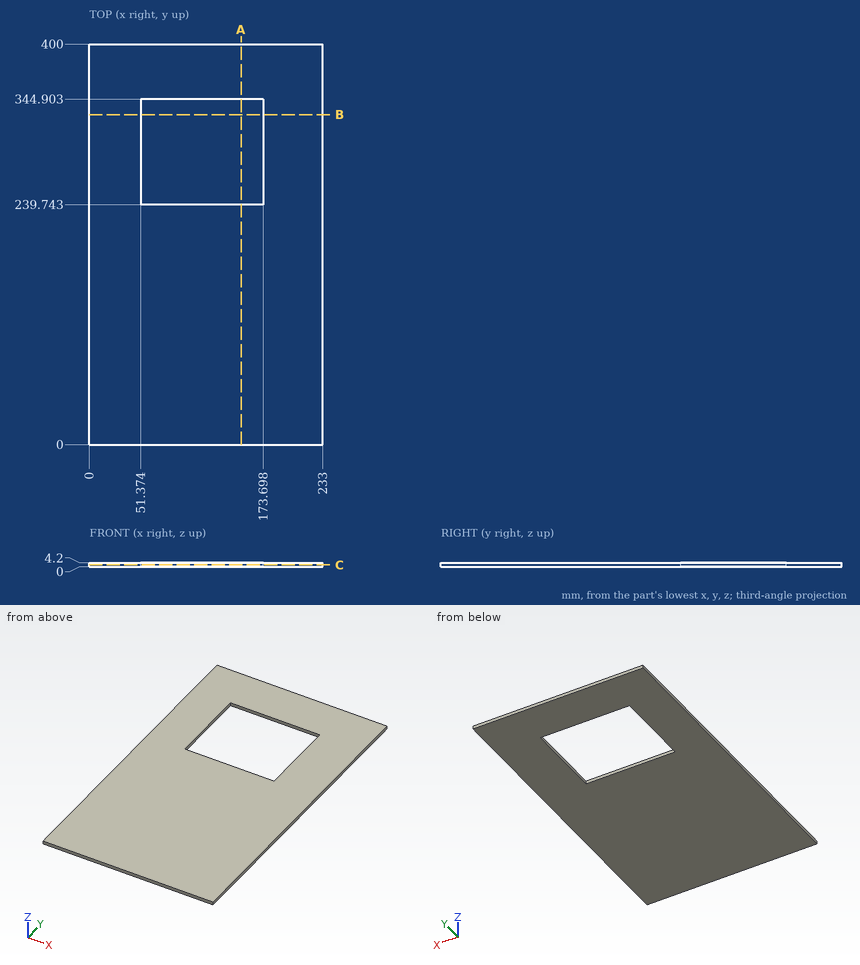
Here's the drawing with two shaded views (mm, measured from the low corner). I have some questions. Coordinates: 2 decimals unless noted, no trailing zeros. Write each loop counter-clockwise with the first axis right and the second up, starting at its lowest first coordinate (ties: lowest second). Pieces come first, ordered by that corner, then holes. Notation, with made-up numbers: (-9.75, 11.25) - (12.25, 11.25) arc R27 cw to (12.25, 37.25) - close; hole circle Ø7 at (48.5, -39.5). An arc over 180 degrees is marked (long way). Return JSON: item names as keys, results as strings.
Q1. If we section it at B-B (y = 329.5): Please give me the cut outline in (x, z).
Computed values:
{"outline": "(0, 0) - (51.37, 0) - (51.37, 4.2) - (0, 4.2) - close; (173.7, 0) - (233, 0) - (233, 4.2) - (173.7, 4.2) - close"}
Q2. Please list where these lines run through material, in increasing order: L1, parallel to Y at x = 140.5, z = 3.3; L2, parallel to X at y = 290, z = 1.8. Write a range as from..to.
Computed values:
{"L1": "y = 0..239.74, 344.9..400", "L2": "x = 0..51.37, 173.7..233"}
Q3. If we section it at A-A (x = 151.5): Please give me the cut outline in (y, z).
Computed values:
{"outline": "(0, 0) - (239.74, 0) - (239.74, 4.2) - (0, 4.2) - close; (344.9, 0) - (400, 0) - (400, 4.2) - (344.9, 4.2) - close"}
Q4. If we section it at C-C (z = 1.9): Please give me the cut outline in (x, y), then the cut area to 3 significant figures.
Computed values:
{"outline": "(0, 0) - (233, 0) - (233, 400) - (0, 400) - close; hole (51.37, 239.74) - (173.7, 239.74) - (173.7, 344.9) - (51.37, 344.9) - close", "area": "80,300 mm2"}
